Can you work these out from the model? Positions are in its coordinate system, mm. A direction names the side the tool comes from. Give positions to 0.01 mm unless a question says otherwise; leave off trailing zeros. Loops run counter-clockwise (first coordinate to the right, second up) from the corner with the lowest first, then second, coordinate; pieces in that order, holes last.
from build123d import *

# Parameters (mm, degrees)
SKETCH1_R           = 2
BOSS_EXTRUDE1_DEPTH = 4


with BuildPart() as part:
    # Sketch1 → Boss-Extrude1 (new body)
    with BuildSketch(Plane(origin=(0, 0, 0), x_dir=(1, 0, 0), z_dir=(0, 1, 0))):
        Polygon((5, 26), (-5, 26), (-5, 30), (-15, 30), (-15, 26), (-19, 26), (-19, 18), (-15, 18), (-15, 10), (-19, 10), (-19, 2), (-15, 2), (-15, -6), (-19, -6), (-19, -14), (-15, -14), (-15, -22), (-19, -22), (-19, -30), (-15, -30), (-6, -30), (-6, -36), (6, -36), (6, -30), (15, -30), (19, -30), (19, -22), (15, -22), (15, -14), (19, -14), (19, -6), (15, -6), (15, 2), (19, 2), (19, 10), (15, 10), (15, 18), (19, 18), (19, 26), (15, 26), (15, 30), (5, 30), align=None)
        with BuildLine():
            ThreePointArc((-4, -18), (-6, -20), (-8, -18))
            ThreePointArc((-8, -18), (-6, -16), (-4, -18))
        make_face(mode=Mode.SUBTRACT)
        with Locations(Location((-6, -12, 0), (0, 0, 270))):
            Circle(SKETCH1_R, mode=Mode.SUBTRACT)
        with Locations(Location((-6, -6, 0), (0, 0, 270))):
            Circle(SKETCH1_R, mode=Mode.SUBTRACT)
        with BuildLine():
            ThreePointArc((4, -18), (6, -16), (8, -18))
            ThreePointArc((8, -18), (6, -20), (4, -18))
        make_face(mode=Mode.SUBTRACT)
        with Locations(Location((6, -12, 0), (0, 0, 270))):
            Circle(SKETCH1_R, mode=Mode.SUBTRACT)
        with Locations(Location((6, -6, 0), (0, 0, 270))):
            Circle(SKETCH1_R, mode=Mode.SUBTRACT)
        with Locations(Location((-6, 0, 0), (0, 0, 270))):
            Circle(SKETCH1_R, mode=Mode.SUBTRACT)
        with Locations(Location((-6, 6, 0), (0, 0, 270))):
            Circle(SKETCH1_R, mode=Mode.SUBTRACT)
        with Locations(Location((-6, 12, 0), (0, 0, 270))):
            Circle(SKETCH1_R, mode=Mode.SUBTRACT)
        with BuildLine():
            ThreePointArc((-4, 18), (-6, 16), (-8, 18))
            ThreePointArc((-8, 18), (-6, 20), (-4, 18))
        make_face(mode=Mode.SUBTRACT)
        with Locations(Location((6, 0, 0), (0, 0, 270))):
            Circle(SKETCH1_R, mode=Mode.SUBTRACT)
        with Locations(Location((6, 6, 0), (0, 0, 270))):
            Circle(SKETCH1_R, mode=Mode.SUBTRACT)
        with Locations(Location((6, 12, 0), (0, 0, 270))):
            Circle(SKETCH1_R, mode=Mode.SUBTRACT)
        with BuildLine():
            ThreePointArc((4, 18), (6, 20), (8, 18))
            ThreePointArc((8, 18), (6, 16), (4, 18))
        make_face(mode=Mode.SUBTRACT)
    extrude(amount=BOSS_EXTRUDE1_DEPTH)


solid = part.part
(1) Suppose I cut it at D-D on x = 14. List the corners of the cut face in (y, z) for me, plus the area to 3 significant figures.
Returned:
outline: (0, -30) - (4, -30) - (4, 30) - (0, 30) - close
area: 240 mm2
(2) Please list where these lines run through material, in increasing order: probe 1 along X at (y, z) = (2.7, -6); probe 2 along X at (y, z) = (1.55, -12); probe 3 along Z at (x, y) = (-17, 1.05).
Returned:
probe 1: x = -19 to -8, -4 to 4, 8 to 19
probe 2: x = -15 to -8, -4 to 4, 8 to 15
probe 3: z = -26 to -18, -10 to -2, 6 to 14, 22 to 30
(3) Suppose I cut it at C-C on z = -6. List the corners of the cut face in (x, y) for me, plus the area to 3 significant figures.
Returned:
outline: (-19, 0) - (-8, 0) - (-8, 4) - (-19, 4) - close; (-4, 0) - (4, 0) - (4, 4) - (-4, 4) - close; (8, 0) - (19, 0) - (19, 4) - (8, 4) - close
area: 120 mm2
(4) Suppose I cut it at A-A on z = 18. List the corners of the cut face in (x, y) for me, plus the area to 3 significant figures.
Returned:
outline: (-15, 0) - (-8, 0) - (-8, 4) - (-15, 4) - close; (-4, 0) - (4, 0) - (4, 4) - (-4, 4) - close; (8, 0) - (15, 0) - (15, 4) - (8, 4) - close
area: 88.0 mm2
(5) Which directions (+Z, -Z, +X, -X, +Y, -Y) give clear straight access to the entire face, cutting with the end or side of a thin tool? Please do faces 5 (the flat face through (15, 2, 2)), 6 (the flat face through (12, 2, 30)), 7 (the flat face through (-17, 2, -26)).
Returned:
face 5: +X, +Y, -Y
face 6: +Z, +X, +Y, -Y
face 7: -Z, -X, +Y, -Y
(6) Will these pins go through, and if not, where does the flat tip stop? P1, Ø1.2, axis at x = 16, y = 1.5, coming from the +Z side; P2, Ø1, axis at x = 3.5, y = 3.5, coming from the -Z side; P3, Ø3.5, axis at x = 6, z = -12, coming from the +Y side; P4, Ø1.2, axis at y = 1, z = 17.5, coming from the +X side.
Returned:
P1: stops at z = 30
P2: stops at z = -26
P3: passes through
P4: stops at x = 15
(7) Thinking about a two-plate mould opening in X: for faces 1 (the cylindrical face through (-6, 2, -20)), 2 (the flat face through (-19, 2, 26)), 3 (the cylindrical face through (-7.2, 2, -1.6)), 4 (the flat face through (0, 4, 3)), which applies, pulls with the +X half, pulls with the -X half, needs draft (parallel to the pull), parting line crosses it, or undercut?
Returned:
face 1: undercut
face 2: pulls with the -X half
face 3: undercut
face 4: needs draft
(8) Suppose I cut it at B-B on y = 0.6. Give the number of separate pieces and of enclosed holes in the cut face, plus the area to 3 significant figures.
Returned:
separate pieces: 1
enclosed holes: 14
area: 1,910 mm2
